Geometry check sheet. Reference: the model listing, model coordinates, mm. Round coordinates to 2 decimals unless told otherwise and drop trailing zeros. Write each loop counter-clockwise with the first axis right and the second up, starting at its lowest first coordinate (ties: lowest second). Pieces come first, ordered by that corner, then holes. Notation, with made-up numbers: (68.25, -39.5) -> (95.25, -39.5) arc R10 ccw to (95.25, -24.5) -> close; hole circle Ø1 at (53.25, 81.25). An arc over 180 degrees is marked (long way). Put each result on its own line as item: value. Start each with the question number.
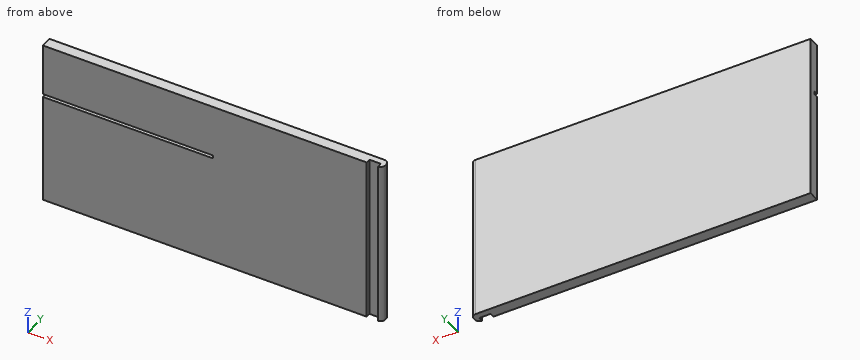
from build123d import *

# Parameters (mm, degrees)
F0_W     = 150
F0_H     = 75
F1_DEPTH = 4.8
F2_W     = 5
F2_H     = 75
F2_W_2   = 75
F2_H_2   = 1.4
F3_DEPTH = 2
F4_R     = 1.99999


# Not quite as in the source:
# - a fillet or chamfer is up to 0.001 mm smaller than in the source, because OpenCascade refuses the exact size


with BuildPart() as f1:
    # F0 (on Front) → F1 (new body)
    with BuildSketch(Plane.XZ):
        Rectangle(F0_W, F0_H)
    extrude(amount=F1_DEPTH)

    # F2 (on face) → F3 (cut)
    with BuildSketch(Plane.XZ.offset(4.8)):
        with Locations((70.5, 0)):
            Rectangle(F2_W, F2_H)
        with Locations((-37.5, 13.2)):
            Rectangle(F2_W_2, F2_H_2)
    extrude(amount=-F3_DEPTH, mode=Mode.SUBTRACT)

    # F4 (radius 2 in the source; OpenCascade refuses exactly that, so slightly less here)
    f4_edges = [f1.edges().sort_by_distance(p)[0] for p in [
        (75, 0, 0),
        (75, -4.8, 0),
    ]]
    fillet(f4_edges, radius=F4_R)


solid = f1.part
(1) Go/stop test with flat-tipped pins: pin 1 Ø1 at (y, z) = (-3.5, 14.5) entering from +X; pin 2 Ø1.5 at (x, z) = (71.5, -16) entering from -Y; pin 3 Ø0.7 at (y, z) = (-4, 13) entering from -X. Record where each tip stops, or that it passes through.
(2) Material ranges on L1, parallel to X at y = -3, z = -32; L2, parallel to Z at x = -42, y = -3.75; L3, parallel to X at y = -3.5, z = 26.5, recorded low to high. Write a range as from..to.
(3) Sectioned sample at A-A (y = -3.55). Record the cut outline in (x, z), and give its area (3 significant figures).
Found:
1. pin 1: x = 74.99
1. pin 2: y = -2.8
1. pin 3: x = 0
2. L1: -75..68, 73..74.99
2. L2: -37.5..12.5, 13.9..37.5
2. L3: -75..68, 73..74.87
3. outline: (-75, -37.5) -> (68, -37.5) -> (68, 37.5) -> (-75, 37.5) -> (-75, 13.9) -> (0, 13.9) -> (0, 12.5) -> (-75, 12.5) -> close; (73, -37.5) -> (74.85, -37.5) -> (74.85, 37.5) -> (73, 37.5) -> close
3. area: 10,800 mm2
